Can you work these out from the model? Positions are in its coordinate system, mm. Face numbers are marked on the shaded views. A direction names the side the tool comes from. Give positions to 0.01 mm unless a question says otherwise; leave off trailing zeros. Write each loop counter-clockwise with the first axis right and the second up, starting at its lowest first coordinate (ties: lowest second). Pieces come first, ordered by that corner, then holes.
1. Suppose I cut it at C-C (y = 17.5). Please give me the cut outline in (x, z), and give its area (3 significant figures).
2. I'm going to push flat-ended pins straight in: pin 1 (10 mm diameter, centred on y = 39, z = 9, fed in from +X); pin 2 (1 mm diameter, centred on y = 8, z = -11.5, fed in from +X); pin 3 (1 mm diameter, centred on x = -39, y = 1, fed in from -Z); pin 4 (1.5 mm diameter, centred on x = 13, y = 7.5, fed in from +Z). Where does each tip first touch, or does it pass through?
3. Suppose I cut it at D-D (z = 8.5). Please give me the cut outline in (x, y), and give its area (3 significant figures).
4. Thinking about a two-plate mould opening in X: for the marked faces 3 and 4, which applies, pulls with the +X half, pulls with the -X half, needs draft (parallel to the pull), parting line crosses it, or undercut?
5. Suppose I cut it at B-B (x = 38). Please give me the cut outline in (y, z), and give its area (3 significant figures).
6. On a 3-axis mill with a long thin cutter (end or side, diameter ignored), from which of +Z, -Z, +X, -X, +Y, -Y can I reach the whole of each face in a straight line? I mean the marked faces 1 and 2. Say none if no direction works.
7. If I drill on probe 1 along X at (y, z) = (0.7, 1.5); probe 2 along X at (y, z) = (6, -3); probe 3 along Z at (x, y) = (38, 1.55), over which ranges is the centre line in solid material (lowest first)?
8. Suppose I cut it at A-A (z = 1.5). Please give me the cut outline in (x, y), and give its area (3 significant figures).
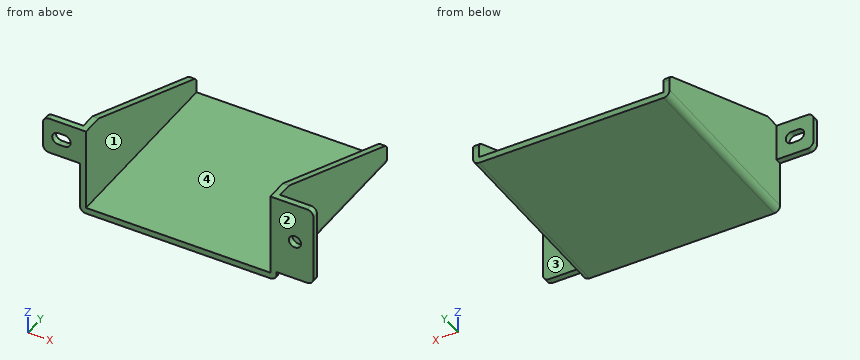
```python
from build123d import *

# Parameters (mm, degrees)
SALIENTE_EXTRUIR1_DEPTH    = 2
SALIENTE_EXTRUIR2_DEPTH    = 60
CORTAR_EXTRUIR1_DEPTH      = 45
CORTAR_EXTRUIR1_DEPTH_BACK = 45
CROQUIS4_R                 = 2
CORTAR_EXTRUIR2_DEPTH      = 3
REDONDEO1_R                = 2


with BuildPart() as part:
    # Croquis1 → Saliente-Extruir1 (new body)
    with BuildSketch(Plane(origin=(0, 0, 0), x_dir=(1, 0, 0), z_dir=(0, 1, 0))):
        Polygon((-32, -2.5), (-32, 14.5), (32, 14.5), (32, 11.5), (44, 11.5), (44, -14.5), (30, -14.5), (30, 12.5), (-30, 12.5), (-30, -14.5), (-44, -14.5), (-44, -2.5), align=None)
    extrude(amount=SALIENTE_EXTRUIR1_DEPTH)

    # Croquis2 → Saliente-Extruir2 (add)
    with BuildSketch(Plane(origin=(0, 2, 0), x_dir=(1, 0, 0), z_dir=(0, 1, 0))):
        Polygon((-32, 14.5), (-32, -2.5), (-32, -14.5), (-30, -14.5), (-30, 12.5), (30, 12.5), (30, -14.5), (32, -14.5), (32, 14.5), align=None)
    extrude(amount=SALIENTE_EXTRUIR2_DEPTH)

    # Croquis3 → Cortar-Extruir1 (cut, two sides)
    with BuildSketch(Plane(origin=(0, 0, 0), x_dir=(0, 0, -1), z_dir=(1, 0, 0))) as cortar_extruir1_sk:
        Polygon((-14.5, 7), (7.5, 62), (-14.5, 62), align=None)
    extrude(amount=CORTAR_EXTRUIR1_DEPTH, mode=Mode.SUBTRACT)
    extrude(cortar_extruir1_sk.sketch, amount=-CORTAR_EXTRUIR1_DEPTH_BACK, mode=Mode.SUBTRACT)

    # Croquis4 → Cortar-Extruir2 (cut, through all)
    with BuildSketch(Plane(origin=(0, 2, 0), x_dir=(1, 0, 0), z_dir=(0, 1, 0))):
        with Locations((38, -1.5)):
            Circle(CROQUIS4_R)
        with BuildLine():
            Line((-39, -6.5), (-37, -6.5))
            ThreePointArc((-37, -6.5), (-35, -8.5), (-37, -10.5))
            Line((-37, -10.5), (-39, -10.5))
            ThreePointArc((-39, -10.5), (-41, -8.5), (-39, -6.5))
        make_face()
    extrude(amount=-CORTAR_EXTRUIR2_DEPTH, mode=Mode.SUBTRACT)

    # Redondeo1
    redondeo1_edges = [part.edges().sort_by_distance(p)[0] for p in [
        (44, 1, -11.5),
        (44, 1, 14.5),
        (-44, 1, 14.5),
        (-44, 1, 2.5),
        (-32, 31, -14.5),
        (32, 31, -14.5),
        (-31, 62, -7.5),
        (31, 62, -7.5),
    ]]
    fillet(redondeo1_edges, radius=REDONDEO1_R)


solid = part.part
```
Checks:
1. outline: (-32, -12.5) arc R2 ccw to (-30, -14.5) - (30, -14.5) arc R2 ccw to (32, -12.5) - (32, 10.3) - (30, 10.3) - (30, -12.5) - (-30, -12.5) - (-30, 10.3) - (-32, 10.3) - close
1. area: 217 mm2
2. pin 1: passes through
2. pin 2: stops at x = 32
2. pin 3: stops at z = 2.5
2. pin 4: stops at z = -12.5
3. outline: (-44, 0) - (-41, 0) - (-41, 2) - (-44, 2) - close; (-35, 0) - (-30, 0) - (-30, 22) - (-32, 22) - (-32, 2) - (-35, 2) - close; (30, 0) - (44, 0) - (44, 2) - (32, 2) - (32, 22) - (30, 22) - close
3. area: 124 mm2
4. face 3: needs draft
4. face 4: undercut
5. outline: (0, -11.5) - (2, -11.5) - (2, -0.5) - (0, -0.5) - close; (0, 3.5) - (2, 3.5) - (2, 14.5) - (0, 14.5) - close
5. area: 44.0 mm2
6. face 1: +Z, +Y, -Y
6. face 2: +Z, -Z, +X, -X, -Y
7. probe 1: x = -32 to -30, 30 to 36, 40 to 44
7. probe 2: x = -32 to -30, 30 to 32
7. probe 3: z = -11.5 to -0.5, 3.5 to 14.5
8. outline: (-32, 0) - (-30, 0) - (-30, 39.5) - (-32, 39.5) - close; (30, 0) - (36, 0) - (36, 2) - (32, 2) - (32, 39.5) - (30, 39.5) - close; (40, 0) - (44, 0) - (44, 2) - (40, 2) - close
8. area: 174 mm2
